The listing builds one solid part. Answer for the finished solid, in the listing's coordinates (mm). A direction names the side the tool comes from. Coordinates: 2 decimals unless noted, no trailing zeros. Order: outer loops, then holes, each group sorted by start corner. A loop starts at its lowest first (then second) coordinate and runs counter-clockwise, first axis right, second up. Notation, with made-up numbers: M 29.5,-2 L 86.5,-2 A13 ccw 86.5,5 Z; hole C 15,19.25 d4. An arc over 180 degrees is marked long. One line per item, written item: value. Start each with the question number.
Q1. Each of these flat-tipped pins is pushed along its axis until it touches: pin 1 Ø1.4 at (y, z) = (41.5, -104.5) entering from -X; pin 2 Ø3 at (x, y) = (-33.5, -43) entering from +Z; pin 3 Ø2.5 at (y, z) = (43, -116) entering from +X; pin 4 Ø8 at (y, z) = (46.5, -27) entering from +X. Where does it stop, or does it pass through?
Q2. The part is cut by section D-D on x = -19.5. Give the vertices of the cut face in (y, z).
Q3. The part is cut by section C-C on x = 0. Give the vertices of the cut face in (y, z) (1 decimal), then the cut area to 3 significant figures.
Q4. The part is cut by section A-A on y = 0. Give the vertices of the cut face in (x, z) (3 decimals), then the cut area to 3 significant figures.
Q5. Determine the mould class of faces 1 (the cylindrical face through (-60.267, 2.652, -125.222)), 2 (the cylindrical face through (1.648, -40.518, -125.222)), 3 (the flat face through (13, -39, -254)) for opening direction X: pulls with the +X half, pulls with the -X half, needs draft (parallel to the pull), parting line crosses it, or undercut.
Q6. For faces 4 (the cylindrical face through (-1.032, 52.438, -230.074)), 5 (the flat face through (0, 44.768, -125)), 6 (the flat face through (13, -39, 0)), determine the directions among +Z, -Z, +X, -X, +Y, -Y from which every point of the face is accessible in a straight line to the end or side of a thin tool.
Q7. Straight lines are drawn through the part: line 1 along Z through (x, y) = (0, 49); line 2 along Y through (x, z) = (1, -195); line 3 along Y through (x, z) = (-15.5, -181). For each, find the intervals that lie inside material, in ascending order. Write a range as [from, to].
```python
from build123d import *

# Parameters (mm, degrees)
F0_R     = 60.325
F1_DEPTH = 254
F2_R     = 4.7625
F3_DEPTH = 60.326
F4_R     = 0.762


with BuildPart() as f1:
    # F0 (on Top) → F1 (new body)
    with BuildSketch(Plane.XY):
        Circle(F0_R)
        with BuildLine():
            ThreePointArc((9.525, 39.416571), (0, -40.5511), (-9.525, 39.416571))
            Line((-9.525, 39.416571), (-9.525, 44.7675))
            Line((-9.525, 44.7675), (9.525, 44.7675))
            Line((9.525, 44.7675), (9.525, 39.416571))
        make_face(mode=Mode.SUBTRACT)
    extrude(amount=-F1_DEPTH)

    # F2 (on Front) → F3 (cut, through all)
    with BuildSketch(Plane.XZ):
        with Locations((0, -28.575)):
            Circle(F2_R)
        with Locations((0, -225.425)):
            Circle(F2_R)
    extrude(amount=-F3_DEPTH, mode=Mode.SUBTRACT)

    # F4
    f4_edges = [f1.edges().sort_by_distance(p)[0] for p in [
        (-9.525, 44.7675, -127),
        (9.525, 44.7675, -127),
    ]]
    fillet(f4_edges, radius=F4_R)


solid = f1.part
```
Output:
1. pin 1: stops at x = -44.43
1. pin 2: stops at z = 0
1. pin 3: stops at x = 43.54
1. pin 4: stops at x = 42.81
2. outline: M -57.09,-254 L -35.55,-254 L -35.55,0 L -57.09,0 Z; M 35.55,-254 L 57.09,-254 L 57.09,0 L 35.55,0 Z
3. outline: M -60.3,-254 L -40.6,-254 L -40.6,0 L -60.3,0 Z; M 44.8,-254 L 60.3,-254 L 60.3,-230.2 L 44.8,-230.2 Z; M 44.8,-220.7 L 60.3,-220.7 L 60.3,-33.3 L 44.8,-33.3 Z; M 44.8,-23.8 L 60.3,-23.8 L 60.3,0 L 44.8,0 Z
3. area: 8,680 mm^2
4. outline: M -60.325,-254 L -40.551,-254 L -40.551,0 L -60.325,0 Z; M 40.551,-254 L 60.325,-254 L 60.325,0 L 40.551,0 Z
4. area: 10,000 mm^2
5. face 1: parting line crosses it
5. face 2: undercut
5. face 3: needs draft
6. face 4: +Y
6. face 5: +Z, -Z
6. face 6: +Z, +X, -X, +Y, -Y
7. line 1: z = [-254, -230.19], [-220.66, -33.34], [-23.81, 0]
7. line 2: y = [-60.32, -40.54], [44.77, 60.32]
7. line 3: y = [-58.3, -37.47], [37.47, 58.3]
